```python
from build123d import *

# Parameters (mm, degrees)
CYLINDER003_R     = 1.5
CYLINDER003_DEPTH = 6
CYLINDER001_R     = 1.5
CYLINDER001_DEPTH = 6
CYLINDER002_R     = 1.5
CYLINDER002_DEPTH = 6
CYLINDER_R        = 1.5
CYLINDER_DEPTH    = 6
BOX001_W          = 50
BOX001_H          = 90
BOX001_DEPTH      = 17
CHAMFER_SIZE      = 3
BOX_W             = 58
BOX_H             = 98
BOX_DEPTH         = 21
FILLET_R          = 3


with BuildPart() as cylinder003:
    # Cylinder003 → Cylinder003 (new body)
    with BuildSketch(Plane(origin=(55.5, 95.5, 15), x_dir=(1, 0, 0), z_dir=(0, 0, 1))):
        Circle(CYLINDER003_R)
    extrude(amount=CYLINDER003_DEPTH)


with BuildPart() as cylinder001:
    # Cylinder001 → Cylinder001 (new body)
    with BuildSketch(Plane(origin=(55.012, 2.02785, 15), x_dir=(1, 0, 0), z_dir=(0, 0, 1))):
        Circle(CYLINDER001_R)
    extrude(amount=CYLINDER001_DEPTH)


with BuildPart() as cylinder002:
    # Cylinder002 → Cylinder002 (new body)
    with BuildSketch(Plane(origin=(2.5, 95.5, 15), x_dir=(1, 0, 0), z_dir=(0, 0, 1))):
        Circle(CYLINDER002_R)
    extrude(amount=CYLINDER002_DEPTH)


with BuildPart() as cylinder:
    # Cylinder → Cylinder (new body)
    with BuildSketch(Plane(origin=(2.5, 2.5, 15), x_dir=(1, 0, 0), z_dir=(0, 0, 1))):
        Circle(CYLINDER_R)
    extrude(amount=CYLINDER_DEPTH)


with BuildPart() as chamfer_body:
    # Box001 → Box001 (new body)
    with BuildSketch(Plane(origin=(4, 4, 4), x_dir=(1, 0, 0), z_dir=(0, 0, 1))):
        with Locations((25, 45)):
            Rectangle(BOX001_W, BOX001_H)
    extrude(amount=BOX001_DEPTH)

    # Chamfer
    chamfer_edges = [chamfer_body.edges().sort_by_distance(p)[0] for p in [
        (4, 49, 4),
        (54, 49, 4),
        (29, 4, 4),
        (29, 94, 4),
    ]]
    chamfer(chamfer_edges, length=CHAMFER_SIZE)


with BuildPart() as case_top:
    # Box → Box (new body)
    with BuildSketch(Plane.XY):
        with Locations((29, 49)):
            Rectangle(BOX_W, BOX_H)
    extrude(amount=BOX_DEPTH)

    # Cut: cut Chamfer body
    add(chamfer_body.part, mode=Mode.SUBTRACT)

    # Fillet
    fillet_edges = [case_top.edges().sort_by_distance(p)[0] for p in [
        (0, 49, 0),
        (29, 0, 0),
        (58, 49, 0),
    ]]
    fillet(fillet_edges, radius=FILLET_R)

    # Cut001: cut Cylinder
    add(cylinder.part, mode=Mode.SUBTRACT)

    # Cut002: cut Cylinder002
    add(cylinder002.part, mode=Mode.SUBTRACT)

    # Cut003: cut Cylinder001
    add(cylinder001.part, mode=Mode.SUBTRACT)

    # Cut004: cut Cylinder003
    add(cylinder003.part, mode=Mode.SUBTRACT)


solid = case_top.part
```
Design review of the part built by this model. Coordinates are the model's own, in mm. A direction names the side the tool comes from. Give positions to 0.01 mm unless a question says otherwise; leave off trailing zeros. Order: outer loops, then holes, each group sorted by start corner. A loop starts at its lowest first (then second) coordinate and runs counter-clockwise, first axis right, second up. Notation, with made-up numbers: M -22.75,47 L -7.75,47 A12 ccw -7.75,70 Z; hole C -24.5,-31.5 d4. An arc over 180 degrees is marked long. One line per question, with ' | ' between items. Start each with the question number.
Q1. We need section C-C (y = 95.5). Write out the cut boundary in (x, z), plus the area to 3 significant figures.
Q2. The part is to be moulded in two halves that separate along X. For faces 1 (the face through (29, 6, 5)), 2 (the face through (57.1, 49.69, 0.86)), 3 (the face through (3, 53, 21)), say which applies: +X half, -X half, draft (parallel to the pull), parting line (faces both ways), or undercut.
Q3. We need section A-A (x = 40.5). Write out the cut boundary in (y, z).
Q4. We need section B-B (z = 10). Write out the cut boundary in (x, y).
Q5. We need section D-D (z = 1.5). Write out the cut boundary in (x, y), plus the area to 3 significant figures.
Q6. For pin 1 Ø1.5 at (x, y) = (56, 95) entering from +Z, flat-tipped, find the tip position at first contact; note if it passes through.
Q7. For L1, parallel to Y at x = 2.5, z = 17.15; L2, parallel to Y at x = 11, z = 8.75; L3, parallel to X at y = 95.5, z = 17, list the stretches that pass through material, from the lowest coordinate up. Write a range as [from, to].
Q8. Machinability: for faces 4 (the face through (29, 51, 0)), 5 (the face through (2.175, 1.036, 17.958)), which of the approach directions +Z, -Z, +X, -X, +Y, -Y give a long, thin tool a straight path to every point of the face, cutting with its end or side? Answer none if there is none.
Returned:
1) outline: M 0,3 A3 ccw 3,0 L 55,0 A3 ccw 58,3 L 58,21 L 57,21 L 57,15 L 54,15 L 54,21 L 4,21 L 4,15 L 1,15 L 1,21 L 0,21 Z | area: 1,180 mm2
2) face 1: undercut | face 2: +X half | face 3: draft
3) outline: M 0,3 A3 ccw 3,0 L 98,0 L 98,21 L 94,21 L 94,7 L 91,4 L 7,4 L 4,7 L 4,21 L 0,21 Z
4) outline: M 0,0 L 58,0 L 58,98 L 0,98 Z; hole M 4,4 L 54,4 L 54,94 L 4,94 Z
5) outline: M 0.4,0.4 L 57.6,0.4 L 57.6,98 L 0.4,98 Z | area: 5,580 mm2
6) pin 1: z = 15
7) L1: [0, 1], [4, 94], [97, 98] | L2: [0, 4], [94, 98] | L3: [0, 1], [4, 54], [57, 58]
8) face 4: -Z, +X, -X, +Y, -Y | face 5: +Z
